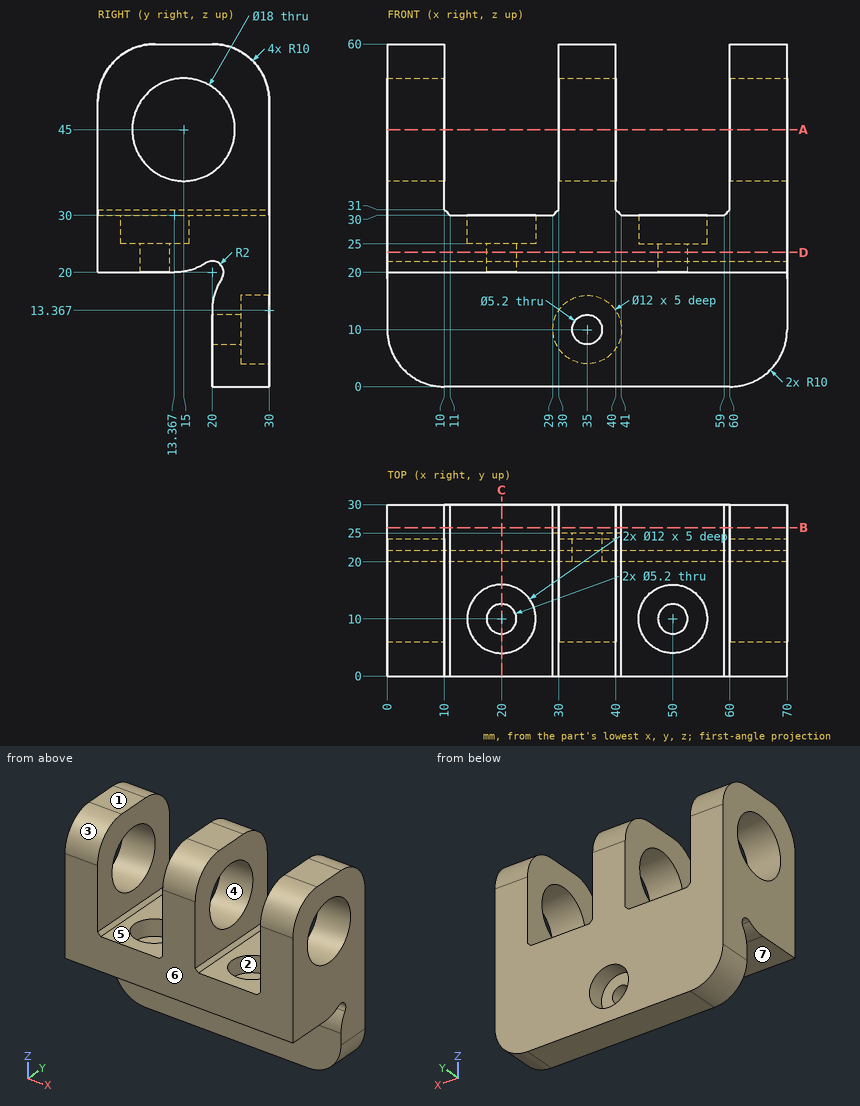
The figure shows three views and two pictorial views of one solid part (mm, origin at its lowest corner). Answer the questions. A direction names the side the tool comes from. Round coordinates to 2 decimals unless told otherwise and drop trailing zeros. Loops run counter-clockwise (first coordinate to the right, second up) from the corner with the lowest first, then second, coordinate; pieces in that order, holes last. Notation, with made-up numbers: M 46.5,30 L 92.5,30 A7 cw 92.5,38 Z; hole C 36,6.5 d6. An arc over 180 degrees is marked long. Return JSON: item names as keys, results as strings.
Q1. Which of the six approach directions +Z, -Z, +X, -X, +Y, -Y give full straight-line access (tool end or side, diameter ignored) to the marked faces 5, 6 and 7?
Results list:
{"face 5": "+Z, +Y, -Y", "face 6": "+Z, -Z, +X, -X, -Y", "face 7": "-Z, +X, -X, -Y"}
Q2. Find section D-D, the plane z = 23.5. Determine the outline of the cut face in (x, y).
Results list:
{"outline": "M 0,0 L 70,0 L 70,30 L 0,30 Z; hole C 20,10 d5.2; hole C 50,10 d5.2"}
Q3. Each of these flat-tipped pins is pushed along its axis until it touches: pin 1 Ø16 at (y, z) = (15, 45) entering from -X; pin 2 Ø5.5 at (x, y) = (47.5, 20) entering from +Z; pin 3 Ø12 at (x, z) = (32.5, 9.5) entering from -Y; pin 4 Ø3 at (x, y) = (32.5, 24) entering from +Z. Where does it stop, or does it pass through?
Results list:
{"pin 1": "passes through", "pin 2": "stops at z = 30", "pin 3": "stops at y = 20", "pin 4": "stops at z = 59.68"}
Q4. Find the intervals of material crossed by line 1 along X through (y, z) = (1.5, 42.5); line 2 along Y through (x, z) = (66, 45); line 3 along Y through (x, z) = (20, 27), in increasing order. Write a range as from..to.
Results list:
{"line 1": "x = 0..10, 30..40, 60..70", "line 2": "y = 0..6, 24..30", "line 3": "y = 0..4, 16..30"}
Q5. Find section C-C, the plane x = 20. Determine the outline of the cut face in (y, z), plus the area to 3 significant figures.
Results list:
{"outline": "M 0,20 L 7.4,20 L 7.4,25 L 4,25 L 4,30 L 0,30 Z; M 12.6,20 L 13.37,20 A10 ccw 18.89,21.67 A2 cw 21.67,18.89 A10 ccw 20,13.37 L 20,0 L 30,0 L 30,30 L 16,30 L 16,25 L 12.6,25 Z", "area": "401 mm2"}
Q6. The mould has two halves that part along Y. Classify the marked faces 1, 2, 3 and 4: released by +Y, released by -Y, zero draft, split by the parting line, or undercut.
Results list:
{"face 1": "zero draft", "face 2": "undercut", "face 3": "released by -Y", "face 4": "undercut"}
Q7. Find section A-A, the plane z = 45. Determine the outline of the cut face in (x, y).
Results list:
{"outline": "M 0,0 L 10,0 L 10,6 L 0,6 Z; M 0,24 L 10,24 L 10,30 L 0,30 Z; M 30,0 L 40,0 L 40,6 L 30,6 Z; M 30,24 L 40,24 L 40,30 L 30,30 Z; M 60,0 L 70,0 L 70,6 L 60,6 Z; M 60,24 L 70,24 L 70,30 L 60,30 Z"}
Q8. Find section B-B, the plane y = 26. Determine the outline of the cut face in (x, z).
Results list:
{"outline": "M 0,10 A10 ccw 10,0 L 60,0 A10 ccw 70,10 L 70,58 L 60,58 L 60,31 L 59,30 L 41,30 L 40,31 L 40,58 L 30,58 L 30,31 L 29,30 L 11,30 L 10,31 L 10,58 L 0,58 Z; hole C 35,10 d12"}
